from build123d import *

# Parameters (mm, degrees)
SKETCH1_R            = 18.5
BOSS_EXTRUDE2_DEPTH  = 20
SKETCH2_R            = 17.25
BOSS_EXTRUDE3_DEPTH  = 30.8
SKETCH3_R            = 1.5
BOSS_EXTRUDE4_DEPTH  = 5
SKETCH5_W            = 1.164728471
SKETCH5_H            = 4.428190706
BOSS_EXTRUDE9_DEPTH  = 8
SKETCH6_R            = 6
BOSS_EXTRUDE12_DEPTH = 6
SKETCH9_R            = 3
BOSS_EXTRUDE13_DEPTH = 15
SKETCH10_W           = 6.033853608
SKETCH10_H           = 1
CUT_EXTRUDE1_DEPTH   = 12
SKETCH11_R           = 1.5
CUT_EXTRUDE4_DEPTH   = 5
CUT_EXTRUDE5_DEPTH   = 0.5
SKETCH13_R           = 17
BOSS_EXTRUDE14_DEPTH = 2.5
SKETCH15_R           = 1.489724088
BOSS_EXTRUDE16_DEPTH = 1
SKETCH16_R           = 7.5
BOSS_EXTRUDE17_DEPTH = 4


# Read off the part's stored shape, not the designer's step: moBlkMgr[GB37]
with BuildPart() as part:
    # Sketch1 → Boss-Extrude2 (new body)
    with BuildSketch(Plane.XY):
        Circle(SKETCH1_R)
    extrude(amount=-BOSS_EXTRUDE2_DEPTH)

    # Sketch2 → Boss-Extrude3 (add)
    with BuildSketch(Plane.XY):
        with Locations(Location((0, 0, 0), (0, 0, 180))):
            Circle(SKETCH2_R)
    extrude(amount=BOSS_EXTRUDE3_DEPTH)

    # Sketch3 → Boss-Extrude4 (add)
    with BuildSketch(Plane.XY.offset(30.8)):
        Circle(SKETCH3_R)
    extrude(amount=BOSS_EXTRUDE4_DEPTH)

    # Sketch5 → Boss-Extrude9 (add)
    with BuildSketch(Plane.XY.offset(30.8)):
        with Locations((14.135311547, 0)):
            Rectangle(SKETCH5_W, SKETCH5_H)
        with Locations((-14.135311547, 0)):
            Rectangle(SKETCH5_W, SKETCH5_H)
    extrude(amount=BOSS_EXTRUDE9_DEPTH)

    # Sketch6 → Boss-Extrude12 (add)
    with BuildSketch(Plane(origin=(0, 0, -20), x_dir=(-1, 0, 0), z_dir=(0, 0, -1))):
        with Locations(Location((0, 7, 0), (0, 0, 180))):
            Circle(SKETCH6_R)
    extrude(amount=BOSS_EXTRUDE12_DEPTH)

    # Sketch9 → Boss-Extrude13 (add)
    with BuildSketch(Plane(origin=(0, 0, -26), x_dir=(-1, 0, 0), z_dir=(0, 0, -1))):
        with Locations((0, 7)):
            Circle(SKETCH9_R)
    extrude(amount=BOSS_EXTRUDE13_DEPTH)

    # Sketch10 → Cut-Extrude1 (cut)
    with BuildSketch(Plane(origin=(0, 0, -41), x_dir=(-1, 0, 0), z_dir=(0, 0, -1))):
        with Locations((0, 9.974859546)):
            Rectangle(SKETCH10_W, SKETCH10_H)
    extrude(amount=-CUT_EXTRUDE1_DEPTH, mode=Mode.SUBTRACT)

    # Sketch11 → Cut-Extrude4 (cut)
    with BuildSketch(Plane(origin=(0, 0, -20), x_dir=(-1, 0, 0), z_dir=(0, 0, -1))):
        with Locations((7.75, 13.423393759)):
            Circle(SKETCH11_R)
        with Locations((15.5, 0)):
            Circle(SKETCH11_R)
        with Locations((7.75, -13.423393759)):
            Circle(SKETCH11_R)
        with Locations((0, -15.5)):
            Circle(SKETCH11_R)
        with Locations((-7.75, -13.423393759)):
            Circle(SKETCH11_R)
        with Locations((-15.5, 0)):
            Circle(SKETCH11_R)
        with Locations((-13.423393759, 7.75)):
            Circle(SKETCH11_R)
        with Locations((-7.75, 13.423393759)):
            Circle(SKETCH11_R)
        with Locations((13.423393759, 7.75)):
            Circle(SKETCH11_R)
    extrude(amount=-CUT_EXTRUDE4_DEPTH, mode=Mode.SUBTRACT)

    # Sketch12 → Cut-Extrude5 (cut)
    with BuildSketch(Plane(origin=(0, 0, -20), x_dir=(-1, 0, 0), z_dir=(0, 0, -1))):
        with BuildLine():
            ThreePointArc((-9.996975987, 5.233316288), (-0.033546899, -11.826522584), (9.929882188, 5.233316288))
            ThreePointArc((9.929882188, 5.233316288), (-0.033546899, -1.867556413), (-9.996975987, 5.233316288))
        make_face()
    extrude(amount=-CUT_EXTRUDE5_DEPTH, mode=Mode.SUBTRACT)

    # Sketch13 → Boss-Extrude14 (add)
    with BuildSketch(Plane.XY.offset(35.8)):
        Circle(SKETCH13_R)
    extrude(amount=-BOSS_EXTRUDE14_DEPTH)

    # Sketch15 → Boss-Extrude16 (add)
    with BuildSketch(Plane.XY.offset(35.8)):
        Circle(SKETCH15_R)
    extrude(amount=BOSS_EXTRUDE16_DEPTH)

    # Sketch16 → Boss-Extrude17 (add)
    with BuildSketch(Plane.XY.offset(36.8)):
        Circle(SKETCH16_R)
    extrude(amount=BOSS_EXTRUDE17_DEPTH)


solid = part.part
Input: part model. Units: mm. Frame: model coordinates. A direction names the side the tool comes from. Coordinates: 2 decimals unless noted, no trailing zeros. Order: outer loops, then holes, each group sorted by start corner. A loop starts at its lowest first (then second) coordinate and runs counter-clockwise, first axis right, second up. Notation, with made-up numbers: M -28,-18 L -24,-18 A19 ccw -24,2 Z; hole C 49.25,8 d9. An arc over 180 degrees is marked long. Write item = value, one per line. Start each with the question number.
(1) Pull-direction query (X, two-part tool) for faces 1 (the cylindrical face through (-0.323, -1.454, 36.293)), 2 (the cylindrical face through (-4.01, -18.06, -9.86)), 3 (the flat face through (0, 7, -41)), 4 (the cylindrical face through (0, -17, -18)); classes: released by +X, released by -X, zero draft, split by the parting line, or undercut.
(2) Section C-C on y = 3. Output: boundary loops of the cut face in (x, z), and give its area (3 significant figures).
(3) Line query: line 1 along Z through (x, y) = (10.5, -4.5); line 2 along Z through (x, y) = (10.5, 8); line 3 along Y through (x, z) = (0, -18.35). Output: solid intervals per line, ascending. Write a range as [from, to].
(4) Section A-A on z = 32.5. Output: boundary loops of the cut face in (x, y), and give its area (3 significant figures).
(5) First-contact query: P1, Ø2, axis at x = 13.5, z = 20, coming from the -Y side; P2, Ø3, axis at y = 10, z = 8, coming from the +X side; P3, Ø12, axis at y = 15, z = 1.5, coming from the -X side. Flat tips, straight axial feed; report the tip coordinate or a pass-through.
(6) Reachability of faces 5 (the flat face through (-8, 13, -15)), 6 (the flat face through (-14.718, 0, 32)), 7 (the flat face through (0, 9.475, -35)), 8 (the flat face through (-13.553, 0, 32)) from +Z, -Z, +X, -X, +Y, -Y: full face, straight path, thin tool, end or side. Return the list, or none.
(7) Section B-B on x = 4. Output: boundary loops of the cut face in (y, z).
(8) Section D-D on z = -17. Give the number of separate pieces and of enclosed holes in the cut face, and give its area (3 significant figures).
Result set:
q1.face_1 = undercut
q1.face_2 = split by the parting line
q1.face_3 = zero draft
q1.face_4 = undercut
q2.outline = M -18.26,-20 L -10.89,-20 L -10.89,-19.5 L -8.85,-19.5 L -8.85,-20 L -4.47,-20 L -4.47,-26 L 4.47,-26 L 4.47,-20 L 8.92,-20 L 8.92,-19.5 L 10.96,-19.5 L 10.96,-20 L 18.26,-20 L 18.26,0 L 16.99,0 L 16.99,30.8 L -16.99,30.8 L -16.99,0 L -18.26,0 Z; M -16.73,33.3 L 16.73,33.3 L 16.73,35.8 L -16.73,35.8 Z; M -6.87,36.8 L 6.87,36.8 L 6.87,40.8 L -6.87,40.8 Z
q2.area = 1,970 mm²
q3.line_1 = [-19.5, 30.8], [33.3, 35.8]
q3.line_2 = [-20, 30.8], [33.3, 35.8]
q3.line_3 = [-18.5, -17], [-14, 18.5]
q4.outline = M -14.72,-2.21 L -13.55,-2.21 L -13.55,2.21 L -14.72,2.21 Z; C 0,0 d3; M 13.55,-2.21 L 14.72,-2.21 L 14.72,2.21 L 13.55,2.21 Z
q4.area = 17.4 mm²
q5.P1 = -11.89
q5.P2 = 15.01
q5.P3 = -16.06
q6.face_5 = -Z
q6.face_6 = -X, +Y, -Y
q6.face_7 = -Z, +X, -X, +Y
q6.face_8 = +Y, -Y
q7.outline = M -18.06,-20 L -11.12,-20 L -11.12,-19.5 L -1.09,-19.5 L -1.09,-20 L 2.53,-20 L 2.53,-26 L 11.47,-26 L 11.47,-20 L 18.06,-20 L 18.06,0 L 16.78,0 L 16.78,30.8 L -16.78,30.8 L -16.78,0 L -18.06,0 Z; M -16.52,33.3 L 16.52,33.3 L 16.52,35.8 L -16.52,35.8 Z; M -6.34,36.8 L 6.34,36.8 L 6.34,40.8 L -6.34,40.8 Z
q8.separate_pieces = 1
q8.enclosed_holes = 9
q8.area = 1,010 mm²
